Read the model definition and answer for the solid it produces. Units are mm, in the model's axes. Face numbers are marked on the shaded views. A direction names the side the tool comes from. Give positions to 0.01 mm unless a question says otherwise; leave off trailing zeros. Order: outer loops, then holes, each group sorted by start corner. A loop starts at its lowest first (then second) coordinate and runs counter-clockwise, first axis right, second up.
```python
from build123d import *

# Parameters (mm, degrees)
F0_R     = 9.5
F1_DEPTH = 2
F2_R     = 8.5
F3_DEPTH = 10
F4_R     = 7.5
F4_R_2   = 7
F5_DEPTH = 10


# Not quite as in the source:
# - a fillet or chamfer that OpenCascade refuses, or shapes differently, is made with other operations: its cross-section is extruded or revolved along the edge and cut away or added


with BuildPart() as f1:
    # F0 (on Right) → F1 (new body)
    with BuildSketch(Plane.YZ):
        Circle(F0_R)
    extrude(amount=F1_DEPTH)

    # F2 (on face) → F3 (join)
    with BuildSketch(Plane.YZ.offset(2)):
        Circle(F2_R)
    extrude(amount=F3_DEPTH)

    # F4 (on face) → F5 (cut)
    with BuildSketch(Plane.YZ.offset(12)):
        Circle(F4_R)
        Circle(F4_R_2, mode=Mode.SUBTRACT)
    extrude(amount=-F5_DEPTH, mode=Mode.SUBTRACT)

    # F6: fillet of radius 4 on 2 edges, made by hand

    # F6_s1 → F6_t2 (revolve, cut)
    with BuildSketch(Plane.XY):
        with BuildLine():
            ThreePointArc((8, 7), (10.8284271247, 5.8284271247), (12, 3))
            Line((12, 3), (12, 7))
            Line((12, 7), (8, 7))
        make_face()
    revolve(axis=Axis((12, 0, 0), (1, 0, 0)), mode=Mode.SUBTRACT)

    # F6_s3 → F6_t4 (revolve, cut)
    with BuildSketch(Plane.XY):
        with BuildLine():
            ThreePointArc((9.3542486889, 8.5), (10.7684622513, 8.2416573868), (12, 7.5))
            Line((12, 7.5), (12, 8.5))
            Line((12, 8.5), (9.3542486889, 8.5))
        make_face()
    revolve(axis=Axis((12, 0, 0), (1, 0, 0)), mode=Mode.SUBTRACT)


solid = f1.part
```
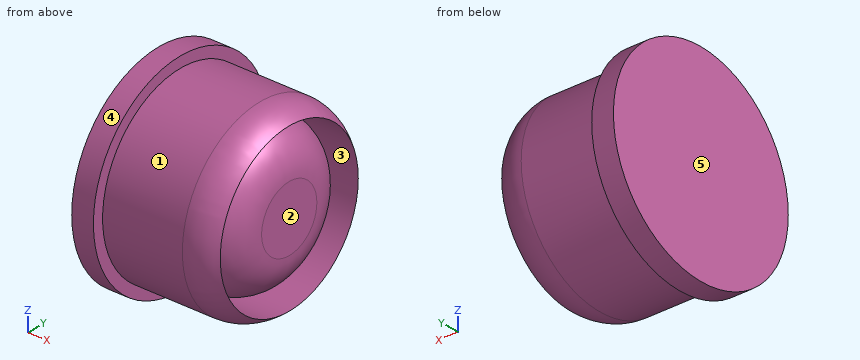
1) The part is cut by section B-B on x = 1.25. Determine the outline of the cut face in (y, z), and give its area (3 significant figures).
Final values:
outline: circle Ø19 at (0, 0)
area: 284 mm2
2) For a pull along Z with two mould halves and no side action, classify the marked faces 3, 4 and 5 as released by +Z, released by -Z, zero draft, split by the parting line, or undercut.
Final values:
face 3: undercut
face 4: split by the parting line
face 5: zero draft
3) Consider L1, parallel to Z at x = 4.25, y = 0; L2, parallel to Y at x = 6.75, z = -1.5; L3, parallel to Y at x = 5, z = 5.75. Determine where each line is inside the solid, lowest interval first.
Final values:
L1: z = -8.5 to -7.5, -7 to 7, 7.5 to 8.5
L2: y = -8.37 to -7.35, -6.84 to 6.84, 7.35 to 8.37
L3: y = -6.26 to -4.82, -3.99 to 3.99, 4.82 to 6.26
4) Given pin 1 (6 mm diameter, centred on x = 9, z = 3, fed in from -Y); pin 2 (3 mm diameter, centred on x = 6.5, y = -1, fed in from +Z); pin 3 (7.5 mm diameter, centred on y = 2.5, z = -3, fed in from +X); pin 4 (2 mm diameter, centred on x = 10, z = -4, fed in from +Y), each flat-ended and moving along its own axis, determine where each tip first touches the part or whether it passes through.
Final values:
pin 1: stops at y = -8.5
pin 2: stops at z = 8.5
pin 3: stops at x = 12
pin 4: stops at y = 7.92
5) A tool of negligible diameter and unlimited length cuts with its end or side. For the marked faces 1 and 2, from which of +Z, -Z, +X, -X, +Y, -Y can it reach the whole face along a straight path? Write none if from no direction.
Final values:
face 1: +X
face 2: +Z, -Z, +X, +Y, -Y
6) The part is cut by section A-A on x = 3.5. Determine the outline of the cut face in (y, z).
Final values:
outline: circle Ø17 at (0, 0); circle Ø14 at (0, 0); hole circle Ø15 at (0, 0)
